from build123d import *

# Parameters (mm, degrees)
ESQUISSE1_W             = 114.5
ESQUISSE1_H             = 64
BOSS_EXTRU_1_DEPTH      = 30.5
ENL_V_MAT_EXTRU_2_DEPTH = 1.5
ESQUISSE3_W             = 111.5
ESQUISSE3_H             = 61
ENL_V_MAT_EXTRU_3_DEPTH = 27.5
ENL_V_MAT_EXTRU_4_REACH = 96.168
ESQUISSE2_4_R           = 1.6
CONG_1_R                = 2
CONG_2_R                = 1


with BuildPart() as part:
    # Esquisse1 → Boss.-Extru.1 (new body)
    with BuildSketch(Plane.XY):
        with Locations((-21.215258856, 10.196525886)):
            Rectangle(ESQUISSE1_W, ESQUISSE1_H)
    extrude(amount=BOSS_EXTRU_1_DEPTH)

    # Esquisse2 → Enl_v. mat.-Extru.2 (cut)
    with BuildSketch(Plane.XY.offset(30.5)):
        with BuildLine():
            ThreePointArc((27.034741144, -20.303474114), (29.231440286, -15.000173256), (34.534741144, -12.803474114))
            Line((34.534741144, -12.803474114), (34.534741144, 33.196525886))
            ThreePointArc((34.534741144, 33.196525886), (29.231440286, 35.393225027), (27.034741144, 40.696525886))
            Line((27.034741144, 40.696525886), (-69.465258856, 40.696525886))
            ThreePointArc((-69.465258856, 40.696525886), (-71.661957997, 35.393225027), (-76.965258856, 33.196525886))
            Line((-76.965258856, 33.196525886), (-76.965258856, -12.803474114))
            ThreePointArc((-76.965258856, -12.803474114), (-71.661957997, -15.000173256), (-69.465258856, -20.303474114))
            Line((-69.465258856, -20.303474114), (27.034741144, -20.303474114))
        make_face()
    extrude(amount=-ENL_V_MAT_EXTRU_2_DEPTH, mode=Mode.SUBTRACT)

    # Esquisse3 → Enl_v. mat.-Extru.3 (cut)
    with BuildSketch(Plane.XY.offset(29)):
        with Locations((-21.215258856, 10.196525886)):
            Rectangle(ESQUISSE3_W, ESQUISSE3_H)
    extrude(amount=-ENL_V_MAT_EXTRU_3_DEPTH, mode=Mode.SUBTRACT)

    # Esquisse2_4 → Enl_v. mat.-Extru.4 (cut, up to next)
    with BuildSketch(Plane.XY.offset(30.5), mode=Mode.PRIVATE) as enl_v_mat_extru_4_sk1:
        with Locations((-73.515258856, 37.246525886)):
            Circle(ESQUISSE2_4_R)
    enl_v_mat_extru_4_tool1 = extrude(enl_v_mat_extru_4_sk1.sketch, amount=-ENL_V_MAT_EXTRU_4_REACH, mode=Mode.PRIVATE) & part.part
    # Esquisse2_4 → Enl_v. mat.-Extru.4 (cut, up to next)
    with BuildSketch(Plane.XY.offset(30.5), mode=Mode.PRIVATE) as enl_v_mat_extru_4_sk2:
        with Locations((31.084741144, -16.853474114)):
            Circle(ESQUISSE2_4_R)
    enl_v_mat_extru_4_tool2 = extrude(enl_v_mat_extru_4_sk2.sketch, amount=-ENL_V_MAT_EXTRU_4_REACH, mode=Mode.PRIVATE) & part.part
    # Esquisse2_4 → Enl_v. mat.-Extru.4 (cut, up to next)
    with BuildSketch(Plane.XY.offset(30.5), mode=Mode.PRIVATE) as enl_v_mat_extru_4_sk3:
        with Locations((-73.515258856, -16.853474114)):
            Circle(ESQUISSE2_4_R)
    enl_v_mat_extru_4_tool3 = extrude(enl_v_mat_extru_4_sk3.sketch, amount=-ENL_V_MAT_EXTRU_4_REACH, mode=Mode.PRIVATE) & part.part
    # Esquisse2_4 → Enl_v. mat.-Extru.4 (cut, up to next)
    with BuildSketch(Plane.XY.offset(30.5), mode=Mode.PRIVATE) as enl_v_mat_extru_4_sk4:
        with Locations((31.084741144, 37.246525886)):
            Circle(ESQUISSE2_4_R)
    enl_v_mat_extru_4_tool4 = extrude(enl_v_mat_extru_4_sk4.sketch, amount=-ENL_V_MAT_EXTRU_4_REACH, mode=Mode.PRIVATE) & part.part
    add(enl_v_mat_extru_4_tool1.solids().sort_by_distance((-73.515259, 37.246526, 30.5))[0], mode=Mode.SUBTRACT)
    add(enl_v_mat_extru_4_tool2.solids().sort_by_distance((31.084741, -16.853474, 30.5))[0], mode=Mode.SUBTRACT)
    add(enl_v_mat_extru_4_tool3.solids().sort_by_distance((-73.515259, -16.853474, 30.5))[0], mode=Mode.SUBTRACT)
    add(enl_v_mat_extru_4_tool4.solids().sort_by_distance((31.084741, 37.246526, 30.5))[0], mode=Mode.SUBTRACT)

    # Cong_1
    cong_1_edges = [part.edges().sort_by_distance(p)[0] for p in [
        (-21.215258856, -21.803474114, 0),
        (-78.465258856, 10.196525886, 0),
        (-21.215258856, 42.196525886, 0),
        (36.034741144, 10.196525886, 0),
        (36.034741144, -21.803474114, 15.25),
        (-78.465258856, -21.803474114, 15.25),
        (-78.465258856, 42.196525886, 15.25),
        (36.034741144, 42.196525886, 15.25),
    ]]
    fillet(cong_1_edges, radius=CONG_1_R)

    # Cong_2
    cong_2_edges = [part.edges().sort_by_distance(p)[0] for p in [
        (-76.965258856, 10.196525886, 1.5),
        (-76.965258856, -20.303474114, 15.25),
        (-21.215258856, 40.696525886, 1.5),
        (-76.965258856, 40.696525886, 15.25),
        (34.534741144, 10.196525886, 1.5),
        (34.534741144, 40.696525886, 15.25),
        (-21.215258856, -20.303474114, 1.5),
        (34.534741144, -20.303474114, 15.25),
    ]]
    fillet(cong_2_edges, radius=CONG_2_R)


solid = part.part
CAD build for the part. Positions are in the model's coordinates, mm. A direction names the side the tool comes from. Give positions to 0.01 mm unless a question says otherwise; leave off trailing zeros. Order: outer loops, then holes, each group sorted by start corner. A loop starts at its lowest first (then second) coordinate and runs counter-clockwise, first axis right, second up. Notation, with made-up numbers: (-31, 34) -> (25, 34) arc R35 cw to (25, 66) -> close; hole circle Ø1 at (-8, 80.5). An arc over 180 degrees is marked (long way). Return JSON: item names as keys, results as strings.
Q1. Flat gauge pin, fed straight in: pin 1 (2.5 mm diameter, centred on x = 31.08, y = 37.25, fed in from +Z). Where does the tip first touch, or does it go through?
Working result:
{"pin 1": "z = 1.5"}
Q2. Saw through at C-C (y = -0.5). Write the cut outline in (x, z), then the cut area to 3 significant figures.
Working result:
{"outline": "(-78.47, 2) arc R2 ccw to (-76.47, 0) -> (34.03, 0) arc R2 ccw to (36.03, 2) -> (36.03, 30.5) -> (34.53, 30.5) -> (34.53, 2.5) arc R1 cw to (33.53, 1.5) -> (-75.97, 1.5) arc R1 cw to (-76.97, 2.5) -> (-76.97, 30.5) -> (-78.47, 30.5) -> close", "area": "257 mm²"}
Q3. Drill centre lines: line 1 (Y direction, x = -51.5, z = 3.5); line 2 (X direction, y = 33, z = 23.5); line 3 (Z direction, x = 23.5, y = -0.5). Where is each one in solid material? Low to high.
Working result:
{"line 1": "-21.8 to -20.3, 40.7 to 42.2", "line 2": "-78.47 to -76.97, 34.53 to 36.03", "line 3": "0 to 1.5"}
Q4. Mould opens along Y. For faces 1 (the face through (-22, -21.803, 16)), 2 (the face through (-78.465, 10, 16)), 3 (the face through (-22, 42.197, 16)), 4 (the face through (-74.785, 36.273, 29.76)) say: pulls with the +Y half, pulls with the -Y half, needs draft (parallel to the pull), parting line crosses it, or undercut.
Working result:
{"face 1": "pulls with the -Y half", "face 2": "needs draft", "face 3": "pulls with the +Y half", "face 4": "undercut"}
Q5. Which spindle directions (+Z, -Z, +X, -X, +Y, -Y) get a long thin tool onto all of the face, cutting with end or side? Do faces 5 (the face through (-22, 11, 0)), 6 (the face through (29.17, -15.06, 29.76)), 7 (the face through (34.535, 10, 17)). Say none if no direction does.
Working result:
{"face 5": "-Z, +X, -X, +Y, -Y", "face 6": "+Z", "face 7": "none"}
Q6. Saw through at B-B (x = -55). Write the cut outline in (y, z).
Working result:
{"outline": "(-21.8, 2) arc R2 ccw to (-19.8, 0) -> (40.2, 0) arc R2 ccw to (42.2, 2) -> (42.2, 30.5) -> (40.7, 30.5) -> (40.7, 2.5) arc R1 cw to (39.7, 1.5) -> (-19.3, 1.5) arc R1 cw to (-20.3, 2.5) -> (-20.3, 30.5) -> (-21.8, 30.5) -> close"}
Q7. Saw through at A-A (z = 16). Write the cut outline in (x, y), then the cut area to 3 significant figures.
Working result:
{"outline": "(-78.47, -19.8) arc R2 ccw to (-76.47, -21.8) -> (34.03, -21.8) arc R2 ccw to (36.03, -19.8) -> (36.03, 40.2) arc R2 ccw to (34.03, 42.2) -> (-76.47, 42.2) arc R2 ccw to (-78.47, 40.2) -> close; hole (-76.97, -19.3) arc R1 ccw to (-75.97, -20.3) -> (33.53, -20.3) arc R1 ccw to (34.53, -19.3) -> (34.53, 39.7) arc R1 ccw to (33.53, 40.7) -> (-75.97, 40.7) arc R1 ccw to (-76.97, 39.7) -> close", "area": "524 mm²"}
